Can you work these out from the drawing? Everything is in mm from the part's minimum corner. A direction names the side the tool comes from. Round coordinates to 2 decimals unless told otherwise and drop trailing zeros. Order: outer loops, then holes, each group sorted by start corner. A loop starts at its lowest first (then second) coordinate and runs counter-clockwise, first axis right, second up. Notation, with made-up numbers: M 75,78.25 L 93,78.25 A29 ccw 93,114.25 Z; hole C 52,-11 d10. An arc over 180 degrees is marked long. Write item = value, one per line. Start each with the question number.
Item 1: For the marked faces 4 and 5, which set-ups out of +Z, -Z, +X, -X, +Y, -Y let a thin tool reach every point of the face, with its end or its side?
Item 2: We'd pull the mould along X, two halves only. Please class the marked faces 1, 2 and 3: pulls with the +X half, pulls with the -X half, needs draft (parallel to the pull), parting line crosses it, or undercut.
Item 3: I'm going to push flat-ended pins straight in: P1, Ø4.5, axis at x = 12.7, y = 44.45, coming from the -Z side; P2, Ø1, axis at x = 11.5, z = 2, coming from the -Y side. Where does each tip first touch, or does it pass through?
Item 4: Please list where these lines run through material, in increasing order: L1, parallel to X at y = 12.7, z = 2.3; L2, parallel to X at y = 13, z = 2.4 (1 decimal).
Item 5: I want a section at B-B, the plane x = 44.45. List the corners of the cut face in (y, z) for me (1 decimal).
Item 6: I want a section at A-A, the plane y = 12.7. List the corners of the cut face in (x, z) for me (1 decimal).
Item 7: I want a section at C-C, the plane z = 2. State how many separate pieces and enclosed holes the cut face has, plus the area to 3 significant figures.
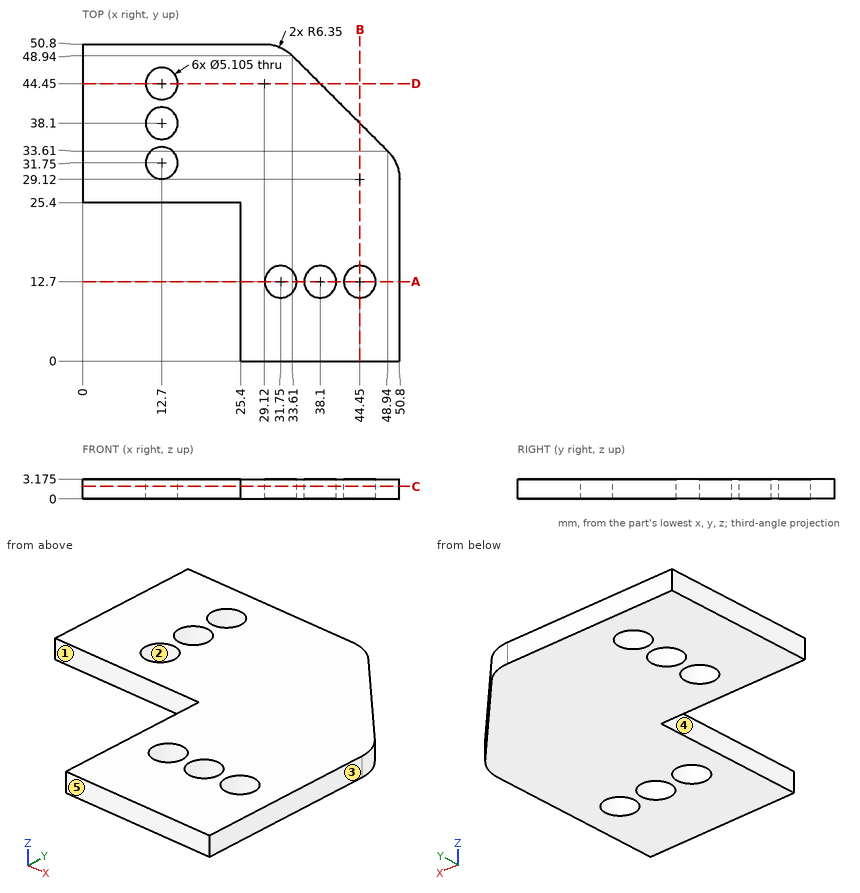
Filled in:
q1.face_4 = +Z, -Z, -X, -Y
q1.face_5 = +Z, -Z, +X, -X, -Y
q2.face_1 = needs draft
q2.face_2 = undercut
q2.face_3 = pulls with the +X half
q3.P1 = through
q3.P2 = 25.4
q4.L1 = 25.4 to 29.2, 34.3 to 35.55, 40.65 to 41.9, 47 to 50.8
q4.L2 = 25.4 to 29.2, 34.3 to 35.6, 40.6 to 41.9, 47 to 50.8
q5.outline = M 0,0 L 10.1,0 L 10.1,3.2 L 0,3.2 Z; M 15.3,0 L 38.1,0 L 38.1,3.2 L 15.3,3.2 Z
q6.outline = M 25.4,0 L 29.2,0 L 29.2,3.2 L 25.4,3.2 Z; M 34.3,0 L 35.5,0 L 35.5,3.2 L 34.3,3.2 Z; M 40.7,0 L 41.9,0 L 41.9,3.2 L 40.7,3.2 Z; M 47,0 L 50.8,0 L 50.8,3.2 L 47,3.2 Z
q7.separate_pieces = 1
q7.enclosed_holes = 6
q7.area = 1,630 mm^2
